CAD build for the part. Positions are in the model's coordinates, mm. Face numbers are marked on the shaded views. A direction names the side the tool comes from. Round coordinates to 2 decimals unless told otherwise and drop trailing zeros. Loops run counter-clockwise (first coordinate to the right, second up) from the corner with the lowest first, then second, coordinate; pieces in that order, holes last.
from build123d import *

# Parameters (mm, degrees)
F1_DEPTH = 63.5
F0_W     = 25.4
F0_H     = 25.4
F2_DEPTH = 19.05
F4_DEPTH = 12.7
F5_R     = 6.35


with BuildPart() as f1:
    # F0 (on Front) → F1 (new body, symmetric)
    with BuildSketch(Plane.XZ):
        Polygon((-50.8, 12.7), (-50.8, -12.7), (50.8, -12.7), (50.8, 12.7), (25.4, 12.7), align=None)
    extrude(amount=F1_DEPTH, both=True)

    # F0 (on Front) → F2 (join, symmetric)
    with BuildSketch(Plane.XZ):
        with BuildLine():
            Line((25.4, 12.7), (50.8, 12.7))
            Line((50.8, 12.7), (50.8, 41.2740438906))
            ThreePointArc((50.8, 41.2740438906), (53.3553304038, 47.7662954815), (59.6502531694, 50.7751144469))
            Line((59.6502531694, 50.7751144469), (82.55, 50.7751144469))
            Line((82.55, 50.7751144469), (82.55, 76.1751144469))
            Line((82.55, 76.1751144469), (59.0323674039, 76.1751144469))
            ThreePointArc((59.0323674039, 76.1751144469), (35.1764332574, 65.5084247532), (25.4, 41.2740438906))
            Line((25.4, 41.2740438906), (25.4, 12.7))
        make_face()
        with Locations((95.25, 63.4751144469)):
            Rectangle(F0_W, F0_H)
    extrude(amount=F2_DEPTH, both=True)

    # F0 (on Front) → F3 (revolve)
    with BuildSketch(Plane.XZ):
        Polygon((107.95, 87.98056042), (107.95, 76.1751144469), (107.95, 50.7751144469), (107.95, 37.18056042), (133.35, 37.18056042), (133.35, 87.98056042), align=None)
    revolve(axis=Axis((107.95, 0, 62.58056042), (0, 0, 1)))

    # F0 (on Front) → F4 (join, symmetric)
    with BuildSketch(Plane.XZ):
        with BuildLine():
            add(Edge.make_bspline(
                [(-50.8, 12.7), (-50.7150068879, 43.1761480868), (16.0312987864, 76.0926790535), (59.0323674039, 76.1751144469)],
                knots=[0, 0, 0, 0, 126.8551894232, 126.8551894232, 126.8551894232, 126.8551894232], degree=3))
            Line((-50.8, 12.7), (25.4, 12.7))
            Line((25.4, 12.7), (25.4, 41.2740438906))
            ThreePointArc((25.4, 41.2740438906), (35.1764332574, 65.5084247532), (59.0323674039, 76.1751144469))
        make_face()
    extrude(amount=F4_DEPTH, both=True)

    # F5
    f5_edges = [f1.edges().sort_by_distance(p)[0] for p in [
        (50.8, -63.5, 0),
        (-50.8, -63.5, 0),
        (-50.8, 63.5, 0),
        (50.8, 63.5, 0),
    ]]
    fillet(f5_edges, radius=F5_R)


solid = f1.part
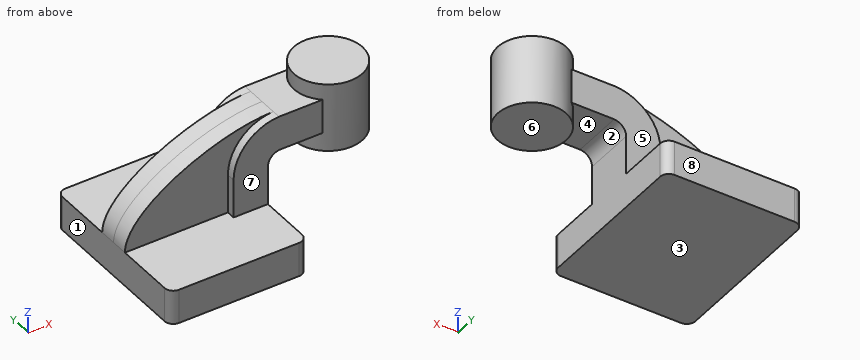
Item 1: Cut at A-A (y = 16). List the corners of the cut face in (x, z) (3 decimals).
Verdict:
outline: (-50.8, -12.7) - (50.8, -12.7) - (50.8, 41.274) arc R9.525 cw to (59.65, 50.775) - (88.223, 50.775) - (88.223, 37.181) - (127.677, 37.181) - (127.677, 87.981) - (88.223, 87.981) - (88.223, 76.175) - (59.032, 76.175) arc R34.925 ccw to (25.4, 41.274) - (25.4, 12.7) - (-50.8, 12.7) - close
Item 2: Wall check: L1, parallel to Z at x = 121, y = -16.5; L2, parallel to Y at x = -12, z = 36; L3, parallel to X at y = -11, z = 4. Give the ranges that are in metal, low to high.
Verdict:
L1: z = 37.18 to 87.98
L2: y = -12.7 to 12.7
L3: x = -50.8 to 50.8
Item 3: Cut at C-C (y = -53.5). List the corners of the cut face in (x, z).
Verdict:
outline: (-50.8, -12.7) - (50.8, -12.7) - (50.8, 12.7) - (-50.8, 12.7) - close
Item 4: Mould opens along X. For the marked faces 1, 2, 3 and 4 say: released by +X, released by -X, zero draft, split by the parting line, or undercut.
Verdict:
face 1: released by -X
face 2: undercut
face 3: zero draft
face 4: undercut
Item 5: Cut at B-B (x = 107.95). List the corners of the cut face in (y, z), plus the area to 3 significant figures.
Verdict:
outline: (-25.4, 37.18) - (25.4, 37.18) - (25.4, 87.98) - (-25.4, 87.98) - close
area: 2,580 mm2
Item 6: Flat gauge pins, fed straight in: P1, Ø7, axis at y = 14.5, z = 34, coming from the -X side; P2, Ø19, axis at x = 8, z = 37, coming from the +Y side; P3, Ø15.5, axis at x = 81, y = -0.5, coming from the -Z side. Where does each tip first touch, or does it go through?
Verdict:
P1: stops at x = -43.47
P2: stops at y = 12.7
P3: stops at z = 37.18
Item 7: 3-axis set-ups, long thin cutter, end or side, ignore diameter. For the marked faces 5, 6, 7 and 8: which of +Z, -Z, +X, -X, +Y, -Y reach the whole face in a straight line?
Verdict:
face 5: +Z, -X, +Y
face 6: -Z, +X, +Y, -Y
face 7: +Z, -X, -Y
face 8: +Z, -Z, +X, -X, +Y
